Build history of the part. All positions in model axes, mm. A direction names the side the tool comes from. Round coordinates to 2 decimals unless told otherwise and drop trailing zeros. Loops run counter-clockwise (first coordinate to the right, second up) from the corner with the lowest first, then second, coordinate; pieces in that order, holes last. Notation, with made-up numbers: (59.25, 29) - (112.25, 29) arc R27 cw to (112.25, 65) - close; hole circle Ø2 at (6, 44). An arc over 180 degrees is marked (long way). Use one line per item in the form item = value. Start each with the question number.
Q1. Saw through at B-B (z = 30). Give the cut face in (x, y).
Q2. Saw through at D-D (y = 16.5). Give the cut face in (x, z).
Q3. Pin check, flat tips, straight feed: pin 1 (8 mm diameter, centred on x = 11, y = -14, fed in from +Z); pin 2 (3 mm diameter, centred on x = 10.5, y = 16, fed in from +Z); pin 3 (3 mm diameter, centred on x = 2, z = 19, fed in from +Y); pin 4 (10 mm diameter, centred on y = 1.5, z = 52, fed in from -X). Stop position of each tip, or through.
Q4. Saw through at A-A (y = 0). Give the cut face in (x, z).
Q5. Saw through at C-C (x = 9). Give the cut face in (y, z).
Q6. 3-axis set-ups, long thin cutter, end or side, ignore diameter. For faces 1 (the face through (0, -30, 30)), 2 (the face through (-7.5, -13, 30)), 3 (the face through (7.5, 13, 30)): which of +Z, -Z, +X, -X, +Y, -Y reach the whole face in a straight line?
Q7. Drill centre lines: line 1 (X direction, y = 25, z = 22.5); line 2 (Y direction, x = 0, z = 40.5); line 3 (Y direction, x = 3, z = 44). Where is each one in solid material? Low to high.
```python
from build123d import *

# Parameters (mm, degrees)
BOSS_EXTRUDE1_DEPTH = 60
SKETCH2_TOOL_BASE_R = 10
BOSS_EXTRUDE2_DEPTH = 20


with BuildPart() as part:
    # sketch1_tool_base → Boss-Extrude1 (new body)
    with BuildSketch(Plane.XY):
        with BuildLine():
            Line((-7.5, 29.047375097), (-7.5, -29.047375097))
            ThreePointArc((-7.5, -29.047375097), (0, -30), (7.5, -29.047375097))
            Line((7.5, -29.047375097), (7.5, 29.047375097))
            ThreePointArc((7.5, 29.047375097), (0, 30), (-7.5, 29.047375097))
        make_face()
    extrude(amount=BOSS_EXTRUDE1_DEPTH)

    # sketch2_tool_base → Boss-Extrude2 (add, symmetric)
    with BuildSketch(Plane(origin=(0, 0, 0), x_dir=(0, 0, -1), z_dir=(1, 0, 0))):
        with Locations((-30, 0)):
            Circle(SKETCH2_TOOL_BASE_R)
    extrude(amount=BOSS_EXTRUDE2_DEPTH, both=True)


solid = part.part
```
Report:
q1.outline = (-20, -10) - (-7.5, -10) - (-7.5, -29.05) arc R30 ccw to (7.5, -29.05) - (7.5, -10) - (20, -10) - (20, 10) - (7.5, 10) - (7.5, 29.05) arc R30 ccw to (-7.5, 29.05) - (-7.5, 10) - (-20, 10) - close
q2.outline = (-7.5, 0) - (7.5, 0) - (7.5, 60) - (-7.5, 60) - close
q3.pin_1 = 60
q3.pin_2 = through
q3.pin_3 = 30
q3.pin_4 = -7.5
q4.outline = (-20, 20) - (-7.5, 20) - (-7.5, 0) - (7.5, 0) - (7.5, 20) - (20, 20) - (20, 40) - (7.5, 40) - (7.5, 60) - (-7.5, 60) - (-7.5, 40) - (-20, 40) - close
q5.outline = circle Ø20 at (0, 30)
q6.face_1 = +Z, -Z, -Y
q6.face_2 = -X
q6.face_3 = +X
q7.line_1 = -7.5 to 7.5
q7.line_2 = -30 to 30
q7.line_3 = -29.85 to 29.85
